Check sheet for the modelled part. Datum: model origin and axes. Units: mm. A direction names the side the tool comes from. Coordinates: 2 decimals unless noted, no trailing zeros. Loops run counter-clockwise (first coordinate to the right, second up) from the corner with the lowest first, then second, coordinate; pieces in that order, holes last. Notation, with made-up numbers: (71.25, -18.5) - (96.25, -18.5) arc R37 ccw to (96.25, 18.5) - close; hole circle Ø1 at (54.25, -7.5). An arc over 180 degrees is marked (long way). Use a Markdown table: item, result. Add a question column.
1) Tool access check on faces 1 (the flat face through (47.75, 12, 0)), 2 (the cylindrical face through (-46.2, 15.1, 14.5)). Record the directions out of +Z, -Z, +X, -X, +Y, -Y that give a thin tool (end or side, any length) a straight path to the whole face; none if there is none.
2) Go/stop test with flat-tipped pins: P1, Ø5.5, axis at x = -44, z = 15, coming from the +Y side; P2, Ø1.5, axis at x = -44.5, z = -15, coming from the +Y side. Record where each tip stops, or that it passes through.
3) Draft check along Z on faces 3 (the flat face through (-1, 25, 0)), 4 (the flat face through (-44, 5, -15)), 5 (the flat face through (-1, 12, -23.5)). Enter one of: pulls with the +Z half, pulls with the -Z half, needs draft (parallel to the pull), parting line crosses it, or undercut.
4) Thickness scan on line 1 (X direction, y = 19.25, z = 15); line 2 (X direction, y = 16.75, z = -17). Record the ranges inside material, lowest first.
5) Sectioned sample at B-B, the plane x = -43.75. Enter the section's corners in (y, z), then the cut area to 3 significant figures.
6) Sectioned sample at A-A, the plane z = -15. Enter the section's corners in (x, y), then the cut area to 3 significant figures.
from build123d import *

# Parameters (mm, degrees)
SKETCH1_W           = 95.5
SKETCH1_H           = 47
BOSS_EXTRUDE1_DEPTH = 25
SKETCH2_R           = 2.5
CUT_EXTRUDE1_DEPTH  = 20
FILLET1_R           = 1


with BuildPart() as part:
    # Sketch1 → Boss-Extrude1 (new body)
    with BuildSketch(Plane(origin=(0, 0, 0), x_dir=(1, 0, 0), z_dir=(0, 1, 0))):
        Rectangle(SKETCH1_W, SKETCH1_H)
    extrude(amount=BOSS_EXTRUDE1_DEPTH)

    # Sketch2 → Cut-Extrude1 (cut)
    with BuildSketch(Plane(origin=(0, 25, 0), x_dir=(1, 0, 0), z_dir=(0, 1, 0))):
        with Locations(Location((-43.75, 15, 0), (0, 0, 270))):
            Circle(SKETCH2_R)
        with Locations(Location((-43.75, -15, 0), (0, 0, 270))):
            Circle(SKETCH2_R)
    extrude(amount=-CUT_EXTRUDE1_DEPTH, mode=Mode.SUBTRACT)

    # Fillet1
    fillet1_edges = [part.edges().sort_by_distance(p)[0] for p in [
        (-47.75, 25, 0),
        (0, 25, 23.5),
        (47.75, 25, 0),
        (0, 0, 23.5),
        (-47.75, 0, 0),
        (0, 0, -23.5),
        (47.75, 0, 0),
        (47.75, 12.5, 23.5),
        (-47.75, 12.5, 23.5),
        (-47.75, 12.5, -23.5),
        (47.75, 12.5, -23.5),
        (0, 25, -23.5),
    ]]
    fillet(fillet1_edges, radius=FILLET1_R)


solid = part.part
Solved:
| question | item | result |
|---|---|---|
| 1 | face 1 | +Z, -Z, +X, +Y, -Y |
| 1 | face 2 | +Y |
| 2 | P1 | stops at y = 25 |
| 2 | P2 | stops at y = 5 |
| 3 | face 3 | needs draft |
| 3 | face 4 | undercut |
| 3 | face 5 | pulls with the -Z half |
| 4 | line 1 | x = -47.75 to -46.25, -41.25 to 47.75 |
| 4 | line 2 | x = -47.75 to -45.25, -42.25 to 47.75 |
| 5 | outline | (0, -22.5) arc R1 ccw to (1, -23.5) - (24, -23.5) arc R1 ccw to (25, -22.5) - (25, -17.5) - (5, -17.5) - (5, -12.5) - (25, -12.5) - (25, 12.5) - (5, 12.5) - (5, 17.5) - (25, 17.5) - (25, 22.5) arc R1 ccw to (24, 23.5) - (1, 23.5) arc R1 ccw to (0, 22.5) - close |
| 5 | area | 974 mm2 |
| 6 | outline | (-47.75, 1) arc R1 ccw to (-46.75, 0) - (46.75, 0) arc R1 ccw to (47.75, 1) - (47.75, 24) arc R1 ccw to (46.75, 25) - (-41.25, 25) - (-41.25, 5) - (-46.25, 5) - (-46.25, 25) - (-46.75, 25) arc R1 ccw to (-47.75, 24) - close |
| 6 | area | 2,290 mm2 |
